The figure shows three views and two pictorial views of one solid part (mm, origin at its lowest corner). Answer the questions. A direction names the side the tool comes from. Round coordinates to 2 decimals unless told otherwise and drop trailing zeros. Order: outer loops, then holes, each group sorted by start corner. A loop starts at its lowest first (then second) coordinate and runs counter-clockwise, first axis right, second up. Notation, with made-up numbers: (-40, 30.5) - (17, 30.5) arc R11 ccw to (17, 50.5) - close; hole circle Ø8 at (-39, 4.5). An arc over 180 degrees is marked (long way). Use CSV: the item, a comma, the result in double quotes.
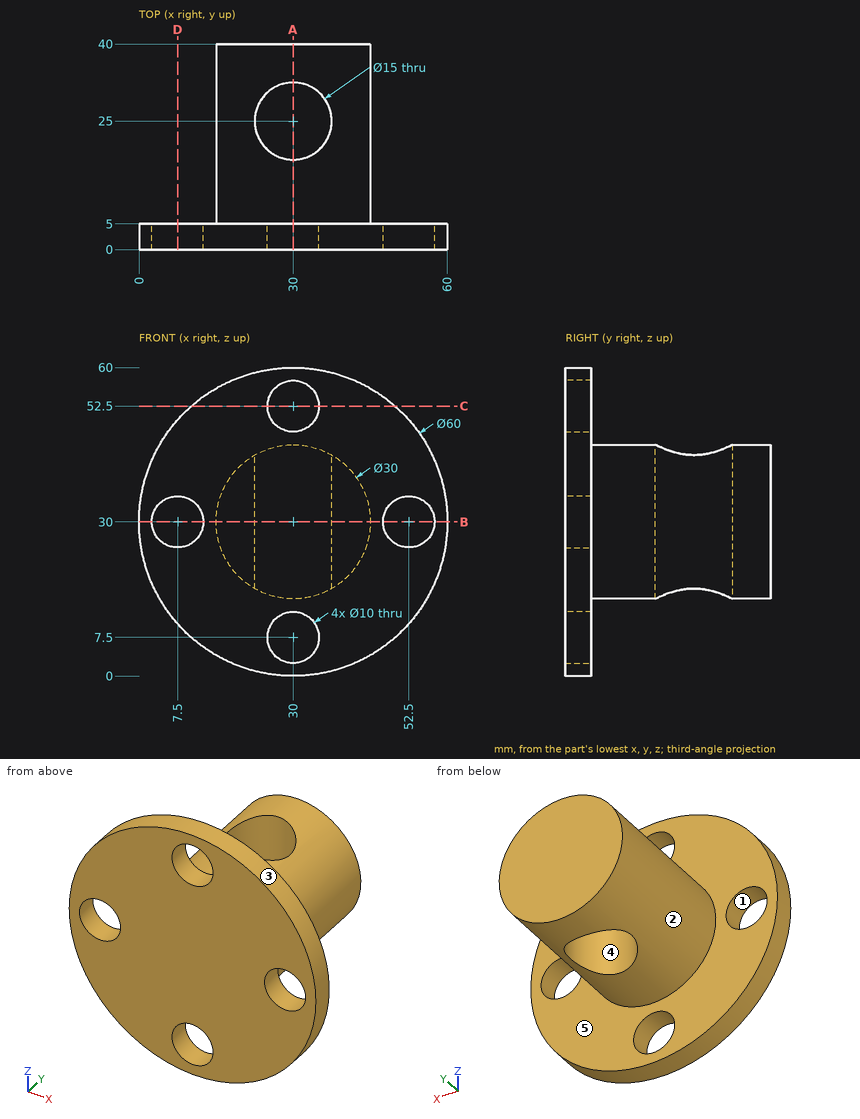
(1) Find section A-A (x = 30). Determine the outline of the cut face in (y, z), and give its area (3 significant figures).
Findings below:
outline,"(0, 0) - (5, 0) - (5, 2.5) - (0, 2.5) - close; (0, 12.5) - (5, 12.5) - (5, 15) - (17.5, 15) - (17.5, 45) - (5, 45) - (5, 47.5) - (0, 47.5) - close; (0, 57.5) - (5, 57.5) - (5, 60) - (0, 60) - close; (32.5, 15) - (40, 15) - (40, 45) - (32.5, 45) - close"
area,"800 mm²"
(2) Find section C-C (z = 52.5). Determine the outline of the cut face in (x, y), and give its area (3 significant figures).
Findings below:
outline,"(10.16, 0) - (25, 0) - (25, 5) - (10.16, 5) - close; (35, 0) - (49.84, 0) - (49.84, 5) - (35, 5) - close"
area,"148 mm²"
(3) Find section D-D (x = 7.5). Determine the outline of the cut face in (y, z), and give its area (3 significant figures).
Findings below:
outline,"(0, 10.16) - (5, 10.16) - (5, 25) - (0, 25) - close; (0, 35) - (5, 35) - (5, 49.84) - (0, 49.84) - close"
area,"148 mm²"
(4) Find section B-B (z = 30). Determine the outline of the cut face in (x, y).
Findings below:
outline,"(0, 0) - (2.5, 0) - (2.5, 5) - (0, 5) - close; (12.5, 0) - (47.5, 0) - (47.5, 5) - (45, 5) - (45, 40) - (15, 40) - (15, 5) - (12.5, 5) - close; (57.5, 0) - (60, 0) - (60, 5) - (57.5, 5) - close; hole circle Ø15 at (30, 25)"
(5) Each of these flat-tipped pins is pushed along its axis until it touches: pin 1 (13 mm diameter, centred on x = 30, z = 7.5, fed in from +Y); pin 2 (1.5 mm diameter, centred on y = 32, z = 27, fed in from +X); pin 3 (5 mm diameter, centred on y = 17.5, z = 24, fed in from +X). Where does it stop, or does it pass through?
Findings below:
pin 1,"stops at y = 5"
pin 2,"stops at x = 44.83"
pin 3,"stops at x = 44.59"
(6) The mould has two halves that part along Y. Classify the marked faces 3, 4 and 5: released by +Y, released by -Y, zero draft, split by the parting line, or undercut.
Findings below:
face 3,"zero draft"
face 4,"undercut"
face 5,"released by +Y"
(7) For the marked faces 1 and 2, determine the directions among +Z, -Z, +X, -X, +Y, -Y from which every point of the face is accessible in a straight line to the end or side of a thin tool.
Findings below:
face 1,"+Y, -Y"
face 2,"+Y"
(8) Find the intervals of material crossed by L1, parallel to X at y = 3, z = 30; L2, parallel to Y at x = 46, z = 14.5; L3, parallel to X at y = 4, z = 9.5, in increasing order. Write a range as from..to.
Findings below:
L1,"x = 0..2.5, 12.5..47.5, 57.5..60"
L2,"y = 0..5"
L3,"x = 8.1..25.42, 34.58..51.9"
